Can you work these out from the drawing? Everything is in mm from the part's minimum corner. A direction names the side the tool comes from. Give positions to 0.01 mm unless a question says otherwise; leave off trailing zeros. Order: outer loops, then holes, each group sorted by start corner. A loop starts at its lowest first (then second) coordinate and runs counter-clockwise, first axis right, second up. Notation, with made-up numbers: M -35.5,39 L -20.5,39 A34 ccw -20.5,75 Z; hole C -5,21 d11. An arc over 180 degrees is marked long. Answer as a JSON object with one key per item and string values.
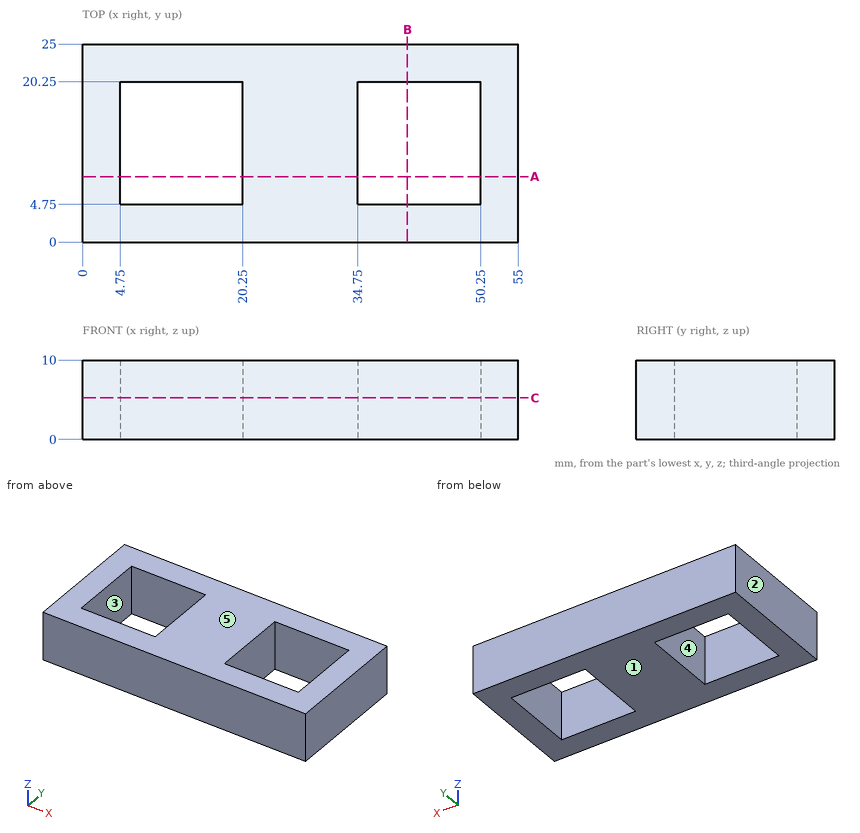
1) I'm going to push a flat-ended pin straight in: pin 1 Ø5 at (x, z) = (41.5, 5.5) entering from -Y. Where does the tip first touch, or does it pass through?
Results found:
{"pin 1": "stops at y = 0"}
2) For the marked faces 4 and 5, which set-ups out of +Z, -Z, +X, -X, +Y, -Y let a thin tool reach every point of the face, with its end or its side?
Results found:
{"face 4": "+Z, -Z", "face 5": "+Z, +X, -X, +Y, -Y"}
3) I want a section at A-A on y = 8.25. Write out the boundary of the cut face in (x, z), and give its area (3 significant figures).
Results found:
{"outline": "M 0,0 L 4.75,0 L 4.75,10 L 0,10 Z; M 20.25,0 L 34.75,0 L 34.75,10 L 20.25,10 Z; M 50.25,0 L 55,0 L 55,10 L 50.25,10 Z", "area": "240 mm²"}
4) I want a section at C-C on z = 5.25. Write out the boundary of the cut face in (x, y).
Results found:
{"outline": "M 0,0 L 55,0 L 55,25 L 0,25 Z; hole M 4.75,4.75 L 20.25,4.75 L 20.25,20.25 L 4.75,20.25 Z; hole M 34.75,4.75 L 50.25,4.75 L 50.25,20.25 L 34.75,20.25 Z"}
5) I want a section at B-B on x = 41. Write out the boundary of the cut face in (y, z), and give its area (3 significant figures).
Results found:
{"outline": "M 0,0 L 4.75,0 L 4.75,10 L 0,10 Z; M 20.25,0 L 25,0 L 25,10 L 20.25,10 Z", "area": "95.0 mm²"}
6) Thinking about a two-plate mould opening in X: for the marked faces 1, 2 and 3, which applies, pulls with the +X half, pulls with the -X half, needs draft (parallel to the pull), parting line crosses it, or undercut?
Results found:
{"face 1": "needs draft", "face 2": "pulls with the -X half", "face 3": "undercut"}
7) I need wall thicknesses on L1, parallel to X at y = 5.5, z = 7.75; L2, parallel to Y at x = 39, z = 1.5. Which ranges of each line are inside material? Lowest first, please.
Results found:
{"L1": "x = 0 to 4.75, 20.25 to 34.75, 50.25 to 55", "L2": "y = 0 to 4.75, 20.25 to 25"}
